Autodesk Inventor part; units mm, degrees
ref_plane "YZ Plane" through (0, 0, 0) normal (1, 0, 0) x (0, 1, 0)
ref_plane "XZ Plane" through (0, 0, 0) normal (0, 1, 0) x (-1, 0, 0)
ref_plane "XY Plane" through (0, 0, 0) normal (0, 0, 1) x (1, 0, 0)
sketch "スケッチ1" plane through (0, 0, 0) normal (0, 0, 1) x (1, 0, 0)
  line L0 (-75, 92) -> (75, 92)
  line L1 (75, 92) -> (75, -92)
  line L2 (75, -92) -> (-75, -92)
  line L3 (-75, -92) -> (-75, 92)
  line L4 (65, 92) -> (65, -92) construction
  line L5 (-65, 92) -> (-65, -92) construction
  line L6 (-65, 0) -> (65, 0) construction
  circle A0 centre (-65, 78) radius 2.25
  circle A1 centre (65, 78) radius 2.25
  circle A2 centre (-65, -78) radius 2.25
  circle A3 centre (65, -78) radius 2.25
  point P0 (0, 0)
  point P1 (0, 92)
  point P2 (-75, 0)
  point P3 (0, 0)
  dimension "d0" = 184
  dimension "d1" = 150
  dimension "d2" = 130
  dimension "d3" = 78
  dimension "d4" = 78
  dimension "d5" = 4.5
extrude "押し出し1" add sketch "スケッチ1" along normal blind 4
sketch "スケッチ3" plane through (0, 0, 0) normal (0, 0, 1) x (1, 0, 0)
  line L0 (-75, -92) -> (75, -92) construction
  line L1 (-75, 92) -> (-75, -92) construction
  line L2 (75, 92) -> (-75, 92) construction
  line L3 (75, -92) -> (75, 92) construction
  circle A0 centre (65, -78) radius 2.25 construction
  circle A1 centre (-65, -78) radius 2.25 construction
  circle A2 centre (65, 78) radius 2.25 construction
  circle A3 centre (-65, 78) radius 2.25 construction
  line L4 (75, 92) -> (-75, 92)
  line L5 (-75, -92) -> (75, -92)
  line L6 (-75, 92) -> (-70, 92)
  line L7 (-70, 92) -> (-70, -92)
  line L8 (-70, -92) -> (-75, -92)
  line L9 (-75, -92) -> (-75, 92)
  line L10 (75, -92) -> (75, 92)
  line L11 (75, 92) -> (70, 92)
  line L12 (70, 92) -> (70, -92)
  line L13 (70, -92) -> (75, -92)
  line L14 (75, -92) -> (75, 92)
  point P0 (0, 0)
  point P1 (70, 92)
  point P2 (70, -92)
  dimension "d8" = 5
extrude "押し出し2" add sketch "スケッチ3" against normal blind 4 contours L10 L5 L12 L4 | L7 L5 L9 L4
sketch "スケッチ4" plane through (0, 0, 0) normal (0, 0, -1) x (-1, 0, 0)
  circle A0 centre (65, 78) radius 2.25 construction
  circle A1 centre (-65, 78) radius 2.25 construction
  circle A2 centre (-65, -78) radius 2.25 construction
  circle A3 centre (65, -78) radius 2.25 construction
  circle A4 centre (65, 78) radius 2.25
  circle A5 centre (65, 78) radius 4.25
  circle A6 centre (65, -78) radius 2.25
  circle A7 centre (65, -78) radius 4.25
  circle A8 centre (-65, 78) radius 2.25
  circle A9 centre (-65, 78) radius 4.25
  circle A10 centre (-65, -78) radius 2.25
  circle A11 centre (-65, -78) radius 4.25
  point P0 (0, 0)
  point P1 (63.9692, 92)
  point P2 (66.0308, 92)
  point P3 (-66.0308, 92)
  point P4 (-63.9692, 92)
  point P5 (-63.9692, -92)
  point P6 (-66.0308, -92)
  point P7 (66.0308, -92)
  point P8 (63.9692, -92)
  dimension "d12" = 8.5
extrude "押し出し3" cut sketch "スケッチ4" against normal blind 1.5 contours A4 | A5 | A6 | A7 | A8 | A9 | A10 | A11
fillet "フィレット1" radius 2 8 edges at (-70, 92, -2) (-75, 92, 0) (70, 92, -2) (75, 92, 0) (75, -92, 0) (70, -92, -2) (-70, -92, -2) (-75, -92, 0)
equation "\"d4\" = d3"
properties part number "bottom_140mm_3"
Check sheet for the modelled part. Datum: model origin and axes. Units: mm. A direction names the side the tool comes from. Give positions to 0.01 mm unless a question says otherwise; leave off trailing zeros. Loops run counter-clockwise (first coordinate to the right, second up) from the corner with the lowest first, then second, coordinate; pieces in that order, holes last. Notation, with made-up numbers: M 5.5,-12 L 54.5,-12 A22 ccw 54.5,16 Z; hole C -14,-2 d5. An arc over 180 degrees is marked long. Answer as a JSON object with one key per item and string values. Group by question number.
Q1. Cross-section at B-B on z = -1.75. Record the cut outline in (x, y).
Q2. Cross-section at D-D on y = -51. Record the cut outline in (x, z).
Q3. Go/stop test with flat-tipped pins: P1, Ø4, axis at x = -67, y = 79.5, coming from the -Z side; P2, Ø1, axis at x = 31.5, z = -1, coming from the -Y side; P3, Ø5, axis at x = 65, y = -78, coming from the -Z side. Record where each tip stops, or that it passes through.
Q4. Cross-section at C-C on y = -78. Record the cut outline in (x, z).
Q5. Material ranges on line 1 along X through (y, z) = (-78, 2.9); line 2 along Y through (x, z) = (-65, 0.8); line 3 along Y through (x, z) = (-65, 3.3), recorded low to high. Write a range as [from, to].
Q6. Cross-section at A-A on x = -65. Record the cut outline in (y, z).
Q7. Access from +Z, -Z, +X, -X, +Y, -Y to the whole of each face (thin tool, end or side, straight path). Record for faces 1 (the cylindrical face through (-65.488, 80.196, 2.732)), 2 (the flat face through (-70, 1, -2)), 3 (the cylindrical face through (-66.96, -81.77, 0.74)).
Evaluation:
{
 "1": {"outline": "M -75,-90 A2 ccw -73,-92 L -72,-92 A2 ccw -70,-90 L -70,90 A2 ccw -72,92 L -73,92 A2 ccw -75,90 Z; M 70,-90 A2 ccw 72,-92 L 73,-92 A2 ccw 75,-90 L 75,90 A2 ccw 73,92 L 72,92 A2 ccw 70,90 Z"},
 "2": {"outline": "M -75,-4 L -70,-4 L -70,0 L 70,0 L 70,-4 L 75,-4 L 75,4 L -75,4 Z"},
 "3": {"P1": "stops at z = 0", "P2": "passes through", "P3": "stops at z = 1.5"},
 "4": {"outline": "M -75,-4 L -70,-4 L -70,0 L -69.25,0 L -69.25,1.5 L -67.25,1.5 L -67.25,4 L -75,4 Z; M -62.75,1.5 L -60.75,1.5 L -60.75,0 L 60.75,0 L 60.75,1.5 L 62.75,1.5 L 62.75,4 L -62.75,4 Z; M 67.25,1.5 L 69.25,1.5 L 69.25,0 L 70,0 L 70,-4 L 75,-4 L 75,4 L 67.25,4 Z"},
 "5": {"line 1": "x = [-75, -67.25], [-62.75, 62.75], [67.25, 75]", "line 2": "y = [-92, -82.25], [-73.75, 73.75], [82.25, 92]", "line 3": "y = [-92, -80.25], [-75.75, 75.75], [80.25, 92]"},
 "6": {"outline": "M -92,0 L -82.25,0 L -82.25,1.5 L -80.25,1.5 L -80.25,4 L -92,4 Z; M -75.75,1.5 L -73.75,1.5 L -73.75,0 L 73.75,0 L 73.75,1.5 L 75.75,1.5 L 75.75,4 L -75.75,4 Z; M 80.25,1.5 L 82.25,1.5 L 82.25,0 L 92,0 L 92,4 L 80.25,4 Z"},
 "7": {"face 1": "+Z, -Z", "face 2": "-Z, +Y, -Y", "face 3": "-Z"}
}
